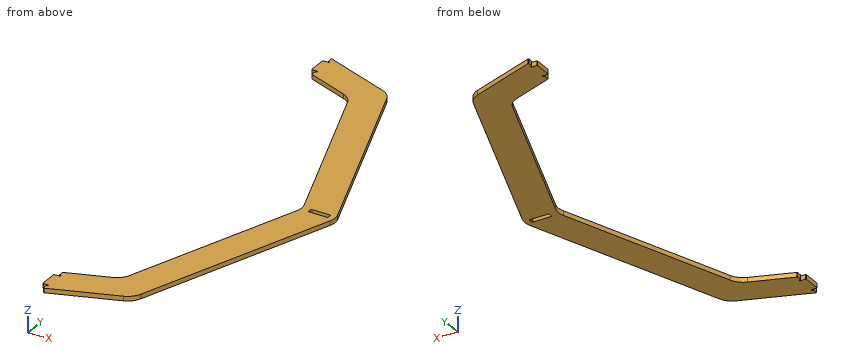
from build123d import *

# Parameters (mm, degrees)
SKETCH1_W           = 13.716
SKETCH1_H           = 3.3528
BOSS_EXTRUDE1_DEPTH = 3.175
FILLET1_R           = 12.7
CUT_EXTRUDE1_DEPTH  = 4.175
FILLET2_R           = 0.508


with BuildPart() as part:
    # Sketch1 → Boss-Extrude1 (new body)
    with BuildSketch(Plane.XY):
        Polygon((114.3, 158.75), (114.3, 146.05), (117.475, 146.05), (117.475, 141.224), (151.477068993, 128.848258983), (198.374, 0), (151.477068993, -128.848258983), (117.475, -141.224), (117.475, -146.05), (114.3, -146.05), (114.3, -158.75), (117.475, -158.75), (117.475, -163.576), (169.035670284, -144.809450758), (221.742, 0), (169.035670284, 144.809450758), (117.475, 163.576), (117.475, 158.75), align=None)
        with Locations((210.058, 0)):
            Rectangle(SKETCH1_W, SKETCH1_H, mode=Mode.SUBTRACT)
    extrude(amount=BOSS_EXTRUDE1_DEPTH)

    # Fillet1
    fillet1_edges = [part.edges().sort_by_distance(p)[0] for p in [
        (169.035670284, 144.809450758, 1.5875),
        (221.742, 0, 1.5875),
        (169.035670284, -144.809450758, 1.5875),
        (151.477068993, -128.848258983, 1.5875),
        (198.374, 0, 1.5875),
        (151.477068993, 128.848258983, 1.5875),
    ]]
    fillet(fillet1_edges, radius=FILLET1_R)

    # Sketch2 → Cut-Extrude1 (cut, through all)
    with BuildSketch(Plane.XY.offset(3.175)):
        with BuildLine():
            Line((117.475, 146.05), (118.237, 146.05))
            ThreePointArc((118.237, 146.05), (118.745, 145.542), (118.237, 145.034))
            Line((118.237, 145.034), (117.475, 145.034))
            Line((117.475, 145.034), (117.475, 146.05))
        make_face()
        with BuildLine():
            Line((117.475, 158.75), (118.237, 158.75))
            ThreePointArc((118.237, 158.75), (118.745, 159.258), (118.237, 159.766))
            Line((118.237, 159.766), (117.475, 159.766))
            Line((117.475, 159.766), (117.475, 158.75))
        make_face()
        with BuildLine():
            Line((117.475, -145.034), (117.475, -146.05))
            Line((117.475, -146.05), (118.237, -146.05))
            ThreePointArc((118.237, -146.05), (118.745, -145.542), (118.237, -145.034))
            Line((118.237, -145.034), (117.475, -145.034))
        make_face()
        with BuildLine():
            Line((117.475, -158.75), (117.475, -159.766))
            Line((117.475, -159.766), (118.237, -159.766))
            ThreePointArc((118.237, -159.766), (118.745, -159.258), (118.237, -158.75))
            Line((118.237, -158.75), (117.475, -158.75))
        make_face()
    extrude(amount=-CUT_EXTRUDE1_DEPTH, mode=Mode.SUBTRACT)

    # Fillet2
    fillet2_edges = [part.edges().sort_by_distance(p)[0] for p in [
        (117.475, 163.576, 1.5875),
        (117.475, -163.576, 1.5875),
        (114.3, -158.75, 1.5875),
        (114.3, -146.05, 1.5875),
        (117.475, -141.224, 1.5875),
        (117.475, 141.224, 1.5875),
        (114.3, 146.05, 1.5875),
        (114.3, 158.75, 1.5875),
        (117.475, 159.766, 1.5875),
        (117.475, -159.766, 1.5875),
        (117.475, -145.034, 1.5875),
        (117.475, 145.034, 1.5875),
        (203.2, 1.6764, 1.5875),
        (203.2, -1.6764, 1.5875),
        (216.916, -1.6764, 1.5875),
        (216.916, 1.6764, 1.5875),
    ]]
    fillet(fillet2_edges, radius=FILLET2_R)


solid = part.part
Geometry check sheet. Reference: the model listing, model coordinates, mm. Give positions to 0.01 mm unless a question says otherwise; leave off trailing zeros. Order: outer loops, then holes, each group sorted by start corner. A loop starts at its lowest first (then second) coordinate and runs counter-clockwise, first axis right, second up.
1. Depth check by flat-ended pin: pin 1 (0.9 mm diameter, centred on y = -142.5, z = 2, fed in from -X) (3 decimals); pin 2 (1 mm diameter, centred on x = 154.5, z = 2, fed in from +Y); pin 3 (1.2 mm diameter, centred on y = 0, z = 1, fed in from -X). Enter the tip coordinate at first touch or a pass-through.
Completed:
pin 1: stops at x = 117.475
pin 2: stops at y = 150.28
pin 3: stops at x = 197.54
2. Scan lines: line 1 (Y direction, x = 133.5, z = 1.8); line 2 (Y direction, x = 139, z = 2.5); line 3 (X direction, y = 3, z = 1.05). Record each from-to range of solid material in increasing order.
Completed:
line 1: y = -157.74 to -135.39, 135.39 to 157.74
line 2: y = -155.74 to -133.39, 133.39 to 155.74
line 3: x = 197.2 to 220.57
3. Sectioned sample at A-A (x = 210). Record the boundary of the cut face in (y, z) (3 decimals), then the cut area to 3 significant figures.
Completed:
outline: (-32.261, 0) - (-1.676, 0) - (-1.676, 3.175) - (-32.261, 3.175) - close; (1.676, 0) - (32.261, 0) - (32.261, 3.175) - (1.676, 3.175) - close
area: 194 mm2
4. Sectioned sample at C-C (y = -37). Record the boundary of the cut face in (x, z) (3 decimals).
Completed:
outline: (184.907, 0) - (208.275, 0) - (208.275, 3.175) - (184.907, 3.175) - close
5. Sectioned sample at B-B (x = 131). Record the boundary of the cut face in (y, z) (3 decimals), then the cut area to 3 significant figures.
Completed:
outline: (-158.653, 0) - (-136.301, 0) - (-136.301, 3.175) - (-158.653, 3.175) - close; (136.301, 0) - (158.653, 0) - (158.653, 3.175) - (136.301, 3.175) - close
area: 142 mm2
